Can you work these out from the model? Positions are in its coordinate system, mm. Face numbers are marked on the shaded views. Coordinates: 2 decimals unless noted, no trailing zeros. Loops run counter-clockwise (first coordinate to the right, second up) from the corner with the lowest first, then second, coordinate; pieces in that order, holes last.
```python
from build123d import *

# Parameters (mm, degrees)
EXTRUDE_START       = 5
EXTRUDE_1_DEPTH     = 5
SKETCH_2_R          = 3
CUT_EXTRUDE_2_DEPTH = 105.040703573


with BuildPart() as part:
    # 草图1 → 凸台-拉伸1 (new body)
    with BuildSketch(Plane(origin=(0, 0, 0), x_dir=(1, 0, 0), z_dir=(0, 1, 0)).offset(EXTRUDE_START)):
        Polygon((17.42, -58.46), (79.42, -66.46), (79.42, -58.46), (17.42, -49.54), align=None)
    extrude(amount=EXTRUDE_1_DEPTH)

    # 草图2 → 切除-拉伸2 (cut, through all)
    with BuildSketch(Plane(origin=(0, 0, 0), x_dir=(1, 0, 0), z_dir=(0, 1, 0))):
        with Locations((18, -54)):
            Circle(SKETCH_2_R)
        with Locations((80, -62)):
            Circle(SKETCH_2_R)
    extrude(amount=CUT_EXTRUDE_2_DEPTH, mode=Mode.SUBTRACT)


solid = part.part
```
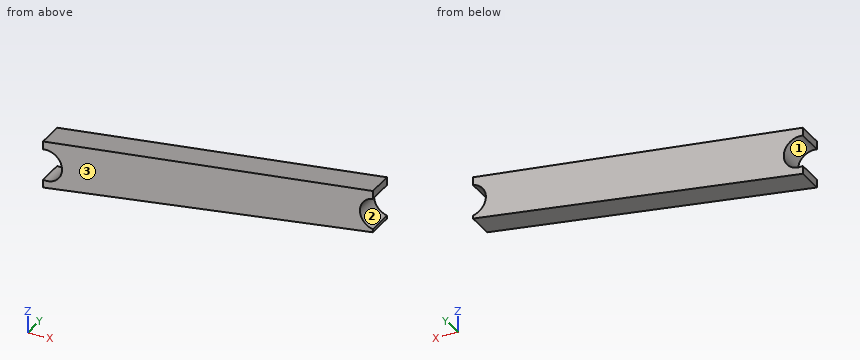
(1) I want a section at D-D on x = 64.5. Write out the boundary of the cut face in (y, z), then the cut area to 3 significant figures.
Check values:
outline: (5, 56.31) - (10, 56.31) - (10, 64.53) - (5, 64.53) - close
area: 41.1 mm2
(2) If I drill on probe 1 along Z at (x, y) = (18, 8.55); probe 2 along Z at (x, y) = (39, 8.8); probe 3 along Z at (x, y) = (58.5, 8.2), over which ranges is the centre line in solid material (lowest first)?
Check values:
probe 1: z = 49.62 to 51, 57 to 58.53
probe 2: z = 52.64 to 61.24
probe 3: z = 55.45 to 63.76
(3) I want a section at B-B on x = 18. Write out the boundary of the cut face in (y, z), then the cut area to 3 significant figures.
Check values:
outline: (5, 49.62) - (10, 49.62) - (10, 51) - (5, 51) - close; (5, 57) - (10, 57) - (10, 58.53) - (5, 58.53) - close
area: 14.6 mm2
(4) I want a section at A-A on y = 6.1. Write out the boundary of the cut face in (x, z), then the cut area to 3 significant figures.
Check values:
outline: (17.42, 49.54) - (79.42, 58.46) - (79.42, 59.06) arc R3 cw to (79.42, 64.94) - (79.42, 66.46) - (17.42, 58.46) - (17.42, 56.94) arc R3 cw (long way) to (17.42, 51.06) - close
area: 496 mm2
(5) I want a section at C-C on z = 54. Write out the boundary of the cut face in (x, y), then the cut area to 3 significant figures.
Check values:
outline: (21, 5) - (48.42, 5) - (48.42, 10) - (21, 10) - close
area: 137 mm2
(6) If we mould it in two halves opening along Z, with no side actions, what happens to the marked faces 1, 2 and 3? For each: released by +Z, released by -Z, zero draft, split by the parting line, or undercut.
Check values:
face 1: undercut
face 2: undercut
face 3: zero draft
